Could you check a few things on this model? Use its own coordinates, in mm. A direction names the side the tool comes from. Give positions to 0.01 mm unless a question says otherwise; leave off trailing zeros. Order: outer loops, then holes, each group sorted by start corner. A loop starts at its lowest first (then second) coordinate and runs counter-clockwise, first axis right, second up. Notation, with made-up numbers: M 32,78.5 L 62,78.5 A18 ccw 62,110.5 Z; hole C 67,45 d2. An arc over 180 degrees is marked long. Answer in a Markdown table with one row per item. Add a question column.
```python
from build123d import *

# Parameters (mm, degrees)
SKETCH1_W           = 15
SKETCH1_H           = 15
BOSS_EXTRUDE1_DEPTH = 170
SKETCH2_R           = 1.75
CUT_EXTRUDE1_DEPTH  = 16
SKETCH8_W           = 15
SKETCH8_H           = 60
BOSS_EXTRUDE2_DEPTH = 50
SKETCH9_W           = 15
SKETCH9_H           = 22
CUT_EXTRUDE2_DEPTH  = 31
SKETCH11_R          = 4.05
CUT_EXTRUDE3_DEPTH  = 10
SKETCH12_W          = 15
SKETCH12_H          = 22
BOSS_EXTRUDE3_DEPTH = 31
CUT_EXTRUDE4_DEPTH  = 16


with BuildPart() as part:
    # Sketch1 → Boss-Extrude1 (new body)
    with BuildSketch(Plane(origin=(0, 0, 0), x_dir=(1, 0, 0), z_dir=(0, 1, 0))):
        Rectangle(SKETCH1_W, SKETCH1_H)
    extrude(amount=BOSS_EXTRUDE1_DEPTH)

    # Sketch2 → Cut-Extrude1 (cut, through all)
    with BuildSketch(Plane(origin=(7.5, 0, 0), x_dir=(0, 0, -1), z_dir=(1, 0, 0))):
        with Locations((0, 9)):
            Circle(SKETCH2_R)
        with Locations((0, 51)):
            Circle(SKETCH2_R)
    extrude(amount=-CUT_EXTRUDE1_DEPTH, mode=Mode.SUBTRACT)

    # Sketch8 → Boss-Extrude2 (add)
    with BuildSketch(Plane(origin=(7.5, 0, 0), x_dir=(0, 0, -1), z_dir=(1, 0, 0))):
        with Locations((0, 140)):
            Rectangle(SKETCH8_W, SKETCH8_H)
    extrude(amount=BOSS_EXTRUDE2_DEPTH)

    # Sketch9 → Cut-Extrude2 (cut)
    with BuildSketch(Plane(origin=(57.5, 0, 0), x_dir=(0, 0, -1), z_dir=(1, 0, 0))):
        with Locations((0, 150)):
            Rectangle(SKETCH9_W, SKETCH9_H)
    extrude(amount=-CUT_EXTRUDE2_DEPTH, mode=Mode.SUBTRACT)

    # Sketch11 → Cut-Extrude3 (cut)
    with BuildSketch(Plane.ZY.offset(7.5)):
        with Locations((0, 161)):
            Circle(SKETCH11_R)
        with Locations((0, 119)):
            Circle(SKETCH11_R)
    extrude(amount=-CUT_EXTRUDE3_DEPTH, mode=Mode.SUBTRACT)

    # Sketch12 → Boss-Extrude3 (add)
    with BuildSketch(Plane(origin=(26.5, 0, 0), x_dir=(0, 0, -1), z_dir=(1, 0, 0))):
        with Locations((0, 150)):
            Rectangle(SKETCH12_W, SKETCH12_H)
    extrude(amount=BOSS_EXTRUDE3_DEPTH)

    # Sketch13 → Cut-Extrude4 (cut, through all)
    with BuildSketch(Plane.XY.offset(7.5)):
        with BuildLine():
            Line((17, 122.8), (7, 122.8))
            ThreePointArc((7, 122.8), (5.3, 124.5), (7, 126.2))
            Line((7, 126.2), (17, 126.2))
            ThreePointArc((17, 126.2), (18.7, 124.5), (17, 122.8))
        make_face()
        with BuildLine():
            Line((32.5, 128.3), (10.8, 128.3))
            ThreePointArc((10.8, 128.3), (-0.9, 140), (10.8, 151.7))
            Line((10.8, 151.7), (32.5, 151.7))
            ThreePointArc((32.5, 151.7), (44.2, 140), (32.5, 128.3))
        make_face()
        with BuildLine():
            Line((48, 122.8), (38, 122.8))
            ThreePointArc((38, 122.8), (36.3, 124.5), (38, 126.2))
            Line((38, 126.2), (48, 126.2))
            ThreePointArc((48, 126.2), (49.7, 124.5), (48, 122.8))
        make_face()
        with BuildLine():
            Line((48, 153.8), (38, 153.8))
            ThreePointArc((38, 153.8), (36.3, 155.5), (38, 157.2))
            Line((38, 157.2), (48, 157.2))
            ThreePointArc((48, 157.2), (49.7, 155.5), (48, 153.8))
        make_face()
        with BuildLine():
            Line((17, 153.8), (7, 153.8))
            ThreePointArc((7, 153.8), (5.3, 155.5), (7, 157.2))
            Line((7, 157.2), (17, 157.2))
            ThreePointArc((17, 157.2), (18.7, 155.5), (17, 153.8))
        make_face()
    extrude(amount=-CUT_EXTRUDE4_DEPTH, mode=Mode.SUBTRACT)


solid = part.part
```
1. Suppose I cut it at A-A on y = 51. List the corners of the cut face in (x, z) for me, plus the area to 4 significant figures.
2. If I drill on line 1 along Y through (x, z) = (48, 3); line 2 along Y through (x, z) = (-5, 0); line 3 along Y through (x, z) = (16.5, -3.75), over which ranges is the centre line in solid material (lowest first)? Write a range as [from, to].
3. For faces 4 (the flat face through (2.5, 161, 0)), 5 (the cylindrical face through (0.11, 49.29, 0.38)), 6 (the flat face through (32, 110, 0)), 7 (the cylindrical face through (-0.897, 139.743, 0.105)), which set-ups out of +Z, -Z, +X, -X, +Y, -Y let a thin tool reach every point of the face, with its end or its side?
4. Suppose I cut it at D-D on x = 13.5. List the corners of the cut face in (y, z) for me, plus the area to 3 significant figures.
5. Will these pins go through, and if not, where does the flat tip stop? P1, Ø2.5, axis at y = 120.5, z = 0.5, coming from the -X side; P2, Ø5, axis at x = 11, z = 1, coming from the -Y side; P3, Ø3, axis at y = 99.5, z = -2, coming from the +X side.
6. Suppose I cut it at B-B on x = -3. List the corners of the cut face in (y, z) for me, plus the area to 3 significant figures.
7. Suppose I cut it at C-C on x = 27. List the corners of the cut face in (y, z) for me.
8. Thinking about a two-plate mould opening in X: for faces 1 (the cylindrical face through (18.7, 124.5, 0.1)), 2 (the flat face through (-7.5, 84, 0)), 3 (the flat face through (17, 122, -7.5)), which applies, pulls with the +X half, pulls with the -X half, needs draft (parallel to the pull), parting line crosses it, or undercut?
Findings below:
| question | item | result |
|---|---|---|
| 1 | outline | M -7.5,-7.5 L 7.5,-7.5 L 7.5,-1.75 L -7.5,-1.75 Z; M -7.5,1.75 L 7.5,1.75 L 7.5,7.5 L -7.5,7.5 Z |
| 1 | area | 172.5 mm2 |
| 2 | line 1 | [110, 122.8], [126.2, 153.8], [157.2, 170] |
| 2 | line 2 | [0, 7.25], [10.75, 49.25], [52.75, 114.95], [123.05, 156.95], [165.05, 170] |
| 2 | line 3 | [110, 122.8], [126.2, 128.3], [151.7, 153.8], [157.2, 170] |
| 3 | face 4 | -X |
| 3 | face 5 | +X, -X |
| 3 | face 6 | +Z, -Z, +X, -Y |
| 3 | face 7 | +Z, -Z |
| 4 | outline | M 110,-7.5 L 122.8,-7.5 L 122.8,7.5 L 110,7.5 Z; M 126.2,-7.5 L 128.3,-7.5 L 128.3,7.5 L 126.2,7.5 Z; M 151.7,-7.5 L 153.8,-7.5 L 153.8,7.5 L 151.7,7.5 Z; M 157.2,-7.5 L 170,-7.5 L 170,7.5 L 157.2,7.5 Z |
| 4 | area | 447 mm2 |
| 5 | P1 | x = 2.5 |
| 5 | P2 | y = 110 |
| 5 | P3 | x = 7.5 |
| 6 | outline | M 0,-7.5 L 170,-7.5 L 170,7.5 L 0,7.5 Z; hole C 9,0 d3.5; hole C 51,0 d3.5; hole C 119,0 d8.1; hole C 161,0 d8.1 |
| 6 | area | 2,430 mm2 |
| 7 | outline | M 110,-7.5 L 128.3,-7.5 L 128.3,7.5 L 110,7.5 Z; M 151.7,-7.5 L 170,-7.5 L 170,7.5 L 151.7,7.5 Z |
| 8 | face 1 | undercut |
| 8 | face 2 | pulls with the -X half |
| 8 | face 3 | needs draft |
